The listing builds one solid part. Answer for the finished solid, in the listing's coordinates (mm). Face numbers are marked on the shaded views. Give positions to 0.01 mm unless a question says otherwise; leave off trailing zeros. Loops run counter-clockwise (first coordinate to the right, second up) from the corner with the lowest first, then second, coordinate; pieces in that order, holes last. Notation, with made-up numbers: (22, -20) - (69, -20) arc R13 cw to (69, -10) - close; hole circle Ø8 at (-16, 72.25). An arc over 180 degrees is marked (long way). Write item = value, one per line. Start each with the question number.
1) Flat-ended cylindrical pins translate along their axes: P1, Ø6, axis at y = 5, z = -23.5, coming from the +X side (3 decimals); P2, Ø5, axis at x = -13, y = 6, coming from the +Z side; P3, Ø3, axis at y = 2, z = -14, coming from the +X side; P4, Ø4, axis at x = 0, z = 0, coming from the +Y side. Find the tip coordinate at first contact, or state that the pin passes through.
2) The part is cut by section B-B on y = 5. Write down the section's boundary in (x, z), plus the area to 3 significant figures.
3) The part is cut by section C-C on z = 0. Write down the section's boundary in (x, y), plus the area to 3 significant figures.
4) The part is cut by section A-A on x = 0. Write down the section's boundary in (y, z), plus the area to 3 significant figures.
5) Consider probe 1 along Y at (x, z) = (17, -4.75); probe 2 along Y at (x, z) = (17, -25); probe 3 along Z at (x, y) = (0, 8.25). Determine where each line is inside the solid, lowest interval first.
6) The part is cut by section D-D on z = -9. Write down the section's boundary in (x, y).
7) The mould has two halves that part along X. Classify the marked faces 1, 2 and 3: +X half, -X half, draft (parallel to the pull), parting line (faces both ways), or undercut.
from build123d import *

# Parameters (mm, degrees)
SKETCH1_R           = 4
BOSS_EXTRUDE1_DEPTH = 10
SKETCH1_3_R         = 4
SKETCH1_3_R_2       = 2.1
BOSS_EXTRUDE2_DEPTH = 11.5
SKETCH1_4_R         = 4
SKETCH1_4_R_2       = 2.1
CUT_EXTRUDE1_DEPTH  = 3.5
SKETCH2_R           = 1.55
CUT_EXTRUDE3_DEPTH  = 61.2
SKETCH3_R           = 51.203530844
SKETCH3_R_2         = 34
CUT_EXTRUDE4_DEPTH  = 56.485642137
SKETCH4_R           = 3
CUT_EXTRUDE5_DEPTH  = 36


with BuildPart() as part:
    # Sketch1 → Boss-Extrude1 (new body)
    with BuildSketch(Plane(origin=(0, 0, 0), x_dir=(1, 0, 0), z_dir=(0, 1, 0))):
        with BuildLine():
            ThreePointArc((1.212086431, -15.076505577), (0, -15.485642137), (-1.212086431, -15.076505577))
            Line((-1.212086431, -15.076505577), (-19.386446667, -1.229373968))
            ThreePointArc((-19.386446667, -1.229373968), (-20.659344965, 0.201570446), (-21.300912355, 2.006082368))
            Line((-21.300912355, 2.006082368), (-27, 40))
            Line((-27, 40), (27, 40))
            Line((27, 40), (21.300912355, 2.006082368))
            ThreePointArc((21.300912355, 2.006082368), (20.659344965, 0.201570446), (19.386446667, -1.229373968))
            Line((19.386446667, -1.229373968), (1.212086431, -15.076505577))
        make_face()
        Circle(SKETCH1_R, mode=Mode.SUBTRACT)
    extrude(amount=BOSS_EXTRUDE1_DEPTH)

    # Sketch1_3 → Boss-Extrude2 (add)
    with BuildSketch(Plane(origin=(0, 0, 0), x_dir=(1, 0, 0), z_dir=(0, 1, 0))):
        Circle(SKETCH1_3_R)
        Circle(SKETCH1_3_R_2, mode=Mode.SUBTRACT)
    extrude(amount=BOSS_EXTRUDE2_DEPTH)

    # Sketch1_4 → Cut-Extrude1 (cut)
    with BuildSketch(Plane(origin=(0, 0, 0), x_dir=(1, 0, 0), z_dir=(0, 1, 0))):
        Circle(SKETCH1_4_R)
        Circle(SKETCH1_4_R_2, mode=Mode.SUBTRACT)
    extrude(amount=CUT_EXTRUDE1_DEPTH, mode=Mode.SUBTRACT)

    # Sketch2 → Cut-Extrude3 (cut)
    with BuildSketch(Plane(origin=(0, 0, -40), x_dir=(-1, 0, 0), z_dir=(0, 0, -1))):
        with Locations((-17, 5)):
            Circle(SKETCH2_R)
        with Locations((17, 5)):
            Circle(SKETCH2_R)
    extrude(amount=-CUT_EXTRUDE3_DEPTH, mode=Mode.SUBTRACT)

    # Sketch3 → Cut-Extrude4 (cut, through all)
    with BuildSketch(Plane(origin=(0, 0, -40), x_dir=(-1, 0, 0), z_dir=(0, 0, -1))):
        with Locations((0, 27.75)):
            Circle(SKETCH3_R)
        with Locations((0, 27.75)):
            Circle(SKETCH3_R_2, mode=Mode.SUBTRACT)
    extrude(amount=-CUT_EXTRUDE4_DEPTH, mode=Mode.SUBTRACT)

    # Sketch4 → Cut-Extrude5 (cut)
    with BuildSketch(Plane(origin=(0, 0, 20), x_dir=(-1, 0, 0), z_dir=(0, 0, -1))):
        with Locations((17, 5)):
            Circle(SKETCH4_R)
        with Locations((-17, 5)):
            Circle(SKETCH4_R)
    extrude(amount=CUT_EXTRUDE5_DEPTH, mode=Mode.SUBTRACT)


solid = part.part
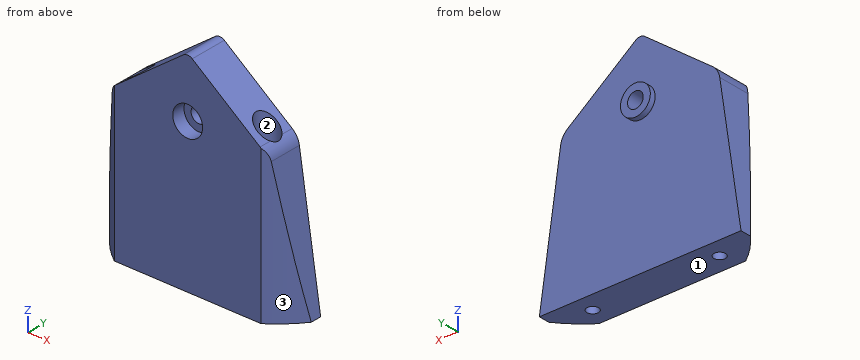
Answer below:
q1.P1 = 24.975
q1.P2 = 8
q1.P3 = 23.27
q1.P4 = through
q2.outline = (-25.27, -40) - (-18.55, -40) - (-18.55, -16) - (-20, -16) - (-20, 0.68) arc R5 ccw to (-21.3, -2.01) - (-25.27, -28.45) - close; (-15.45, -40) - (15.45, -40) - (15.45, -16) - (14, -16) - (14, 5.33) - (1.21, 15.08) arc R2 ccw to (-1.21, 15.08) - (-14, 5.33) - (-14, -16) - (-15.45, -16) - close; (18.55, -40) - (25.27, -40) - (25.27, -28.45) - (21.3, -2.01) arc R5 ccw to (20, 0.68) - (20, -16) - (18.55, -16) - close; hole circle Ø4.2 at (0, 0)
q2.area = 1,840 mm2
q3.outline = (-20.53, 0.65) arc R34 ccw to (-19.65, 0) - (-4, 0) - (-4, 3.5) - (-2.1, 3.5) - (-2.1, 11.5) - (-4, 11.5) - (-4, 10) - (-20.53, 10) - close; (2.1, 3.5) - (4, 3.5) - (4, 0) - (19.65, 0) arc R34 ccw to (20.53, 0.65) - (20.53, 10) - (4, 10) - (4, 11.5) - (2.1, 11.5) - close; hole circle Ø6 at (-17, 5); hole circle Ø6 at (17, 5)
q3.area = 304 mm2
q4.outline = (0, -40) - (10, -40) - (10, -4) - (11.5, -4) - (11.5, -2.1) - (3.5, -2.1) - (3.5, -4) - (0, -4) - close; (0, 4) - (3.5, 4) - (3.5, 2.1) - (11.5, 2.1) - (11.5, 4) - (10, 4) - (10, 15.49) - (0, 15.49) - close
q4.area = 505 mm2
q5.probe_1 = 0 to 2, 8 to 10
q5.probe_2 = 0 to 3.45, 6.55 to 10
q5.probe_3 = -40 to -2.1, 2.1 to 15.49
q6.outline = (-22.35, 2.13) arc R34 ccw to (-19.65, 0) - (19.65, 0) arc R34 ccw to (22.35, 2.13) - (22.35, 10) - (-22.35, 10) - close; hole circle Ø6 at (-17, 5); hole circle Ø6 at (17, 5)
q7.face_1 = draft
q7.face_2 = undercut
q7.face_3 = +X half
